The model under review builds one solid part; all positions refer to its coordinate system, in mm. Face numbers are marked on the shaded views. A direction names the side the tool comes from. Coordinates: 2 decimals unless noted, no trailing zeros. Loops run counter-clockwise (first coordinate to the right, second up) from the corner with the lowest first, then second, coordinate; pieces in that order, holes last. Notation, with made-up numbers: (24, 24) - (46, 24) arc R21 ccw to (46, 53) - close; hole circle Ø5 at (62.25, -13.5). An arc over 180 degrees is marked (long way). One line per item, written item: value. Start each with the question number.
1. We need section D-D, the plane z = -54.5. Give the boundary of the cut face in (x, y), then the cut area to 3 significant figures.
2. Insertion check: P1, Ø1, axis at y = 31, z = -19, coming from the +X side; P2, Ø3, axis at y = 28.5, z = -43, coming from the -X side; P3, Ø5, axis at x = -10, z = -35, coming from the -Y side; P4, Ø5, axis at y = 20, z = -24, coming from the -X side. Each pin has a flat end and moves straight along its axis. Give the tip position at first contact, or say it passes through.
3. For the marked faces 1 and 2, list the 3-axis set-ups (+Z, -Z, +X, -X, +Y, -Y) from which the entire face can be reached by the end or side of a thin tool; tool diameter is ignored.
4. We need section C-C, the plane y = 28. Give the boundary of the cut face in (x, z), then the cut area to 3 significant figures.
5. To check wall thickness, follow line 1 (Z direction, x = -10, y = 8); line 2 (Z direction, x = -12.5, y = 2); line 3 (X direction, y = 21.5, z = -10). State the ranges of each line that lie inside material, in increasing order.
6. We need section A-A, the plane x = -10. Give the boundary of the cut face in (y, z).
7. We need section B-B, the plane z = -10. Give the boundary of the cut face in (x, y), then the cut area to 3 significant figures.
Autodesk Inventor part; units mm, degrees
ref_plane "YZ Plane" through (0, 0, 0) normal (1, 0, 0) x (0, 1, 0)
ref_plane "XZ Plane" through (0, 0, 0) normal (0, 1, 0) x (-1, 0, 0)
ref_plane "XY Plane" through (0, 0, 0) normal (0, 0, 1) x (1, 0, 0)
sketch "Sketch1" plane through (0, 0, 0) normal (0, 1, 0) x (-1, 0, 0)
  line L0 (0, 0) -> (20, 0)
  line L1 (20, 0) -> (20, -70)
  line L2 (20, -70) -> (0, -70)
  line L3 (0, -70) -> (0, 0)
  dimension "d0" = 70
  dimension "d1" = 20
extrude "Extrusion1" add sketch "Sketch1" along normal blind 35
sketch "Sketch2" plane through (0, 35, 0) normal (0, 1, 0) x (1, 0, 0)
  line L0 (-20, 70) -> (-20, 0)
  line L1 (0, 70) -> (-20, 70)
  point P0 (0, 0)
  point P1 (-10, 60)
  point P2 (-20, 35)
  point P3 (-10, 70)
  point P4 (-10, 35)
  point P5 (-10, 10)
  dimension "d5" = 10
  dimension "d6" = 10
  dimension "d14" = 25
  dimension "d15" = 25
hole "Hole1" at (-10, 35, -60) at (-10, 35, -35) at (-10, 35, -10) direction (0, -1, 0) diameter 6 end through all
sketch "Sketch3" plane through (0, 0, -70) normal (0, 0, -1) x (-1, 0, 0)
  line L0 (0, 0) -> (20, 0)
  line L1 (20, 0) -> (20, 20)
  line L2 (20, 0) -> (20, 35)
  line L3 (20, 20) -> (40, 0)
  line L4 (40, 0) -> (20, 0)
  dimension "d16" = 20
  dimension "d17" = 45
extrude "Extrusion2" add sketch "Sketch3" against normal up to surface (70 mm away)
properties part number "Magazine_Mount_Plate_Spacer_3DPrint"
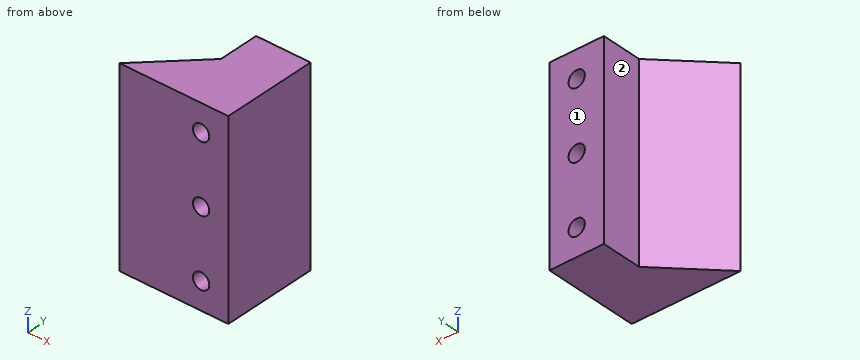
Findings below:
1. outline: (-40, 0) - (0, 0) - (0, 35) - (-20, 35) - (-20, 20) - close
1. area: 900 mm2
2. P1: x = 0
2. P2: x = -20
2. P3: through
2. P4: x = -22.5
3. face 1: +Z, -Z, +X, -X, +Y
3. face 2: +Z, -Z, -X, +Y
4. outline: (-20, -70) - (0, -70) - (0, 0) - (-20, 0) - close; hole circle Ø6 at (-10, -60); hole circle Ø6 at (-10, -35); hole circle Ø6 at (-10, -10)
4. area: 1,320 mm2
5. line 1: -70 to -63, -57 to -38, -32 to -13, -7 to 0
5. line 2: -70 to -61.66, -58.34 to -36.66, -33.34 to -11.66, -8.34 to 0
5. line 3: -20 to -13, -7 to 0
6. outline: (0, -70) - (35, -70) - (35, -63) - (0, -63) - close; (0, -57) - (35, -57) - (35, -38) - (0, -38) - close; (0, -32) - (35, -32) - (35, -13) - (0, -13) - close; (0, -7) - (35, -7) - (35, 0) - (0, 0) - close
7. outline: (-40, 0) - (-13, 0) - (-13, 35) - (-20, 35) - (-20, 20) - close; (-7, 0) - (0, 0) - (0, 35) - (-7, 35) - close
7. area: 690 mm2
